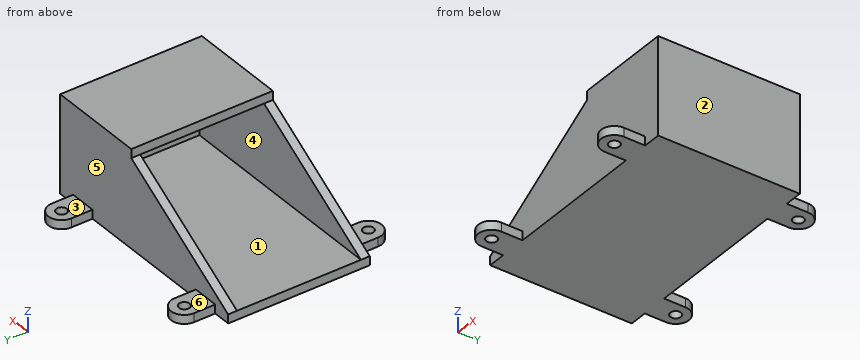
```python
from build123d import *

# Parameters (mm, degrees)
SKETCH_1_W             = 125
SKETCH_1_H             = 70
EXTRUDE_1_DEPTH        = 5
EXTRUDE_2_DEPTH        = 5
PATTERN_LINEAR_1_COUNT = 2
PATTERN_LINEAR_1_PITCH = 75
SKETCH_4_W             = 50
SKETCH_4_H             = 80
EXTRUDE_3_DEPTH        = 5
SKETCH_5_W             = 55
SKETCH_5_H             = 80
EXTRUDE_4_DEPTH        = 5
EXTRUDE_5_DEPTH        = 5
PATTERN_LINEAR_2_COUNT = 2
PATTERN_LINEAR_2_PITCH = 95
MIRROR_1_COPY_1_DEPTH  = 5


with BuildPart() as part:
    # 草圖1 → 填料-伸長1 (new body)
    with BuildSketch(Plane.XY):
        with Locations((62.5, 35)):
            Rectangle(SKETCH_1_W, SKETCH_1_H)
    extrude(amount=EXTRUDE_1_DEPTH)

    # 草圖2 → 填料-伸長2 (add)
    with BuildSketch(Plane.XZ):
        Polygon((75, 50), (0, 5), (0, 0), (125, 0), (125, 50), align=None)
    extrude_2 = extrude(amount=EXTRUDE_2_DEPTH)

    # 直線複製排列1: 填料-伸長2 ×2
    with Locations(*[(0, i * PATTERN_LINEAR_1_PITCH, 0) for i in range(1, PATTERN_LINEAR_1_COUNT)]):
        add(extrude_2)

    # 草圖4 → 填料-伸長3 (add)
    with BuildSketch(Plane(origin=(125, 0, 0), x_dir=(0, 0, -1), z_dir=(1, 0, 0))):
        with Locations((-25, 35)):
            Rectangle(SKETCH_4_W, SKETCH_4_H)
    extrude(amount=EXTRUDE_3_DEPTH)

    # 草圖5 → 填料-伸長4 (add)
    with BuildSketch(Plane.XY.offset(50)):
        with Locations((102.5, 35)):
            Rectangle(SKETCH_5_W, SKETCH_5_H)
    extrude(amount=EXTRUDE_4_DEPTH)

    # 草圖6 → 填料-伸長5 (add)
    with BuildSketch(Plane.XY):
        with BuildLine():
            Line((25, -5), (10, -5))
            Line((10, -5), (10, -17))
            ThreePointArc((10, -17), (17.5, -9.5), (25, -17))
            Line((25, -17), (25, -5))
        make_face()
        with BuildLine():
            ThreePointArc((25, -17), (17.5, -9.5), (10, -17))
            Line((10, -17), (14.5, -17))
            ThreePointArc((14.5, -17), (17.5, -14), (20.5, -17))
            Line((20.5, -17), (25, -17))
        make_face()
        with BuildLine():
            Line((14.5, -17), (10, -17))
            ThreePointArc((10, -17), (17.5, -24.5), (25, -17))
            Line((25, -17), (20.5, -17))
            ThreePointArc((20.5, -17), (17.5, -20), (14.5, -17))
        make_face()
    extrude_5 = extrude(amount=EXTRUDE_5_DEPTH)

    # 直線複製排列2: 填料-伸長5 ×2
    with Locations(*[(i * PATTERN_LINEAR_2_PITCH, 0, 0) for i in range(1, PATTERN_LINEAR_2_COUNT)]):
        add(extrude_5)

    # 鏡射1: 填料-伸長5 across plane
    add(extrude_5.mirror(Plane.ZX.offset(35)))

    # 鏡射1 copy 1 sketch → 鏡射1 copy 1 (add)
    with BuildSketch(Plane(origin=(95, 70, 0), x_dir=(1, 0, 0), z_dir=(0, 0, 1))):
        with BuildLine():
            Line((25, 5), (10, 5))
            Line((10, 5), (10, 17))
            ThreePointArc((10, 17), (17.5, 9.5), (25, 17))
            Line((25, 17), (25, 5))
        make_face()
        with BuildLine():
            ThreePointArc((25, 17), (17.5, 9.5), (10, 17))
            Line((10, 17), (14.5, 17))
            ThreePointArc((14.5, 17), (17.5, 14), (20.5, 17))
            Line((20.5, 17), (25, 17))
        make_face()
        with BuildLine():
            Line((14.5, 17), (10, 17))
            ThreePointArc((10, 17), (17.5, 24.5), (25, 17))
            Line((25, 17), (20.5, 17))
            ThreePointArc((20.5, 17), (17.5, 20), (14.5, 17))
        make_face()
    extrude(amount=MIRROR_1_COPY_1_DEPTH)


solid = part.part
```
Part model, mm, in its own coordinate system. Face numbers are marked on the shaded views. A direction names the side the tool comes from. Give positions to 0.01 mm unless a question says otherwise; leave off trailing zeros. Write each loop counter-clockwise with the first axis right and the second up, starting at its lowest first coordinate (ties: lowest second). Pieces come first, ordered by that corner, then holes. Notation, with made-up numbers: M 85.5,-24 L 89.5,-24 A16 ccw 89.5,-1 Z; hole C 43,-7.5 d6. An arc over 180 degrees is marked long. Use CSV: the item, a comma, the result in double quotes.
Item 1: Slice it at A-A on x = 112.5. Write the cut outline in (y, z).
Taken from the geometry:
outline,"M -24.5,0 L -20,0 L -20,5 L -24.5,5 Z; M -14,0 L 84,0 L 84,5 L 75,5 L 75,55 L -5,55 L -5,5 L -14,5 Z; M 90,0 L 94.5,0 L 94.5,5 L 90,5 Z; hole M 0,5 L 70,5 L 70,50 L 0,50 Z"
Item 2: Slice it at D-D on z = 27. Write the cut outline in (x, y).
Taken from the geometry:
outline,"M 36.67,-5 L 130,-5 L 130,75 L 36.67,75 L 36.67,70 L 125,70 L 125,0 L 36.67,0 Z"
Item 3: Drill centre lines: probe 1 along Y at (x, z) = (112.5, 1.1); probe 2 along X at (y, z) = (-17, 3.5); probe 3 along Z at (x, y) = (103, 37). Where is each one in solid material? Low to high.
Taken from the geometry:
probe 1,"y = -24.5 to -20, -14 to 84, 90 to 94.5"
probe 2,"x = 10 to 14.5, 20.5 to 25, 105 to 109.5, 115.5 to 120"
probe 3,"z = 0 to 5, 50 to 55"
Item 4: Pin check, flat tips, straight feed: P1, Ø10, axis at y = 43, z = 12, coming from the -X side; P2, Ø2.5, axis at y = 79.5, z = 3.5, coming from the -X side; P3, Ø8, axis at x = 62.5, y = 63.5, coming from the -Z side; P4, Ø7.5, axis at x = 111.5, y = 85, coming from the +Z side. Stop position of each tip, or through.
Taken from the geometry:
P1,"stops at x = 125"
P2,"stops at x = 10"
P3,"stops at z = 0"
P4,"stops at z = 5"
Item 5: Pull direction Z, two halves, no side cores. Call the marked faces 4, 5 and 6: +Z half, -Z half, draft (parallel to the pull), parting line (faces both ways), or undercut.
Taken from the geometry:
face 4,"undercut"
face 5,"draft"
face 6,"+Z half"
Item 6: Which spindle directions (+Z, -Z, +X, -X, +Y, -Y) get a long thin tool onto all of the face, cutting with end or side? Do the marked faces 1, 2 and 3. Say none if no direction does.
Taken from the geometry:
face 1,"-X"
face 2,"+Z, -Z, +X, +Y, -Y"
face 3,"+Z, +X, -X, +Y"
Item 7: Slice it at C-C on y = 51. Write the cut outline in (x, z).
Taken from the geometry:
outline,"M 0,0 L 130,0 L 130,55 L 75,55 L 75,50 L 125,50 L 125,5 L 0,5 Z"
Item 8: Slice it at B-B on x = 17.5. Write the cut outline in (y, z).
Taken from the geometry:
outline,"M -24.5,0 L -20,0 L -20,5 L -24.5,5 Z; M -14,0 L 84,0 L 84,5 L 75,5 L 75,15.5 L 70,15.5 L 70,5 L 0,5 L 0,15.5 L -5,15.5 L -5,5 L -14,5 Z; M 90,0 L 94.5,0 L 94.5,5 L 90,5 Z"
